from build123d import *

# Parameters (mm, degrees)
F1_R      = 46
F2_DEPTH  = 8
F3_R      = 39.8466862326
F4_DEPTH  = 6
F7_DEPTH  = 25
F9_ANGLE  = 120
F10_ANGLE = 120
F13_DEPTH = 8
F15_DEPTH = 8
F16_ANGLE = 120
F18_DEPTH = 6
F20_DEPTH = 6
F21_R     = 1
F22_R     = 2
F23_R     = 2


with BuildPart() as f2:
    # F1 (on offset) → F2 (new body)
    with BuildSketch(Plane.XY.offset(-3)):
        Circle(F1_R)
    extrude(amount=F2_DEPTH)


with BuildPart() as f4:
    # F3 (on Top) → F4 (new body)
    with BuildSketch(Plane.XY):
        Circle(F3_R)
    extrude(amount=F4_DEPTH)


with BuildPart() as f2_1:
    add(f2.part)

    # F5: cut F4
    add(f4.part, mode=Mode.SUBTRACT)


with BuildPart() as f7:
    # F6 (on Top) → F7 (new body)
    with BuildSketch(Plane.XY):
        Polygon((4.2, 46.7533776755), (-4.2, 46.7533776755), (-5, 38), (5, 38), align=None)
    extrude(amount=F7_DEPTH)


with BuildPart() as f9_1:
    # F9: copy of F7
    add(f7.part.rotate(Axis((0, 0, 3.5398988872), (0, 0, -1)), F9_ANGLE))


with BuildPart() as f10_1:
    # F10: copy of F9_1
    add(f9_1.part.rotate(Axis((0, 0, 3.5398988872), (0, 0, -1)), F10_ANGLE))


with BuildPart() as f2_2:
    add(f2_1.part)

    # F11: cut F10_1, F9_1, F7
    add(f10_1.part, mode=Mode.SUBTRACT)
    add(f9_1.part, mode=Mode.SUBTRACT)
    add(f7.part, mode=Mode.SUBTRACT)



with BuildPart() as f13:
    # F12 (on offset) → F13 (new body)
    with BuildSketch(Plane.XY.offset(-3)):
        Polygon((1.9, 49.994420498), (-1.9, 49.925893195), (-3, 36.9057094163), (3, 36.9057094163), align=None)
    extrude(amount=F13_DEPTH)


with BuildPart() as f15:
    # F14 (on offset) → F15 (new body)
    with BuildSketch(Plane.XY.offset(-3)):
        Polygon((42.1813093126, -26.4778193086), (44.179931283, -23.2300590724), (28.5657010972, -12.1127264574), (24.8182862997, -18.1085914373), align=None)
    extrude(amount=F15_DEPTH)


with BuildPart() as f16_1:
    # F16: copy of F15
    add(f15.part.rotate(Axis((0, 0, 3.5398988872), (0, 0, -1)), F16_ANGLE))


with BuildPart() as f18:
    # F17 (on Top) → F18 (new body)
    with BuildSketch(Plane.XY):
        Polygon((25.2, 21.096765488), (12.9, 34.6466732368), (-12.9, 34.6466732368), (-25.2, 21.096765488), (-24.2, 6.7315296738), (-30.2, 5.9), (-30.2, -2.6), (-25.2, -4.6), (-21, -5.2), (-21, 3.5), (-3.3, -0.8), (3.3, -0.8), (21, 3.5), (21, -5.2), (25.2, -4.6), (30.2, -2.5974751513), (30.2, 5.9025248487), (24.2, 6.7315296738), align=None)
    extrude(amount=F18_DEPTH)


with BuildPart() as f2_3:
    add(f2_2.part)

    add(f13.part)  # F20 merges F13

    add(f15.part)  # F20 merges F15

    add(f16_1.part)  # F20 merges F16_1

    add(f18.part)  # F20 merges F18
    # F19 (on Top) → F20 (join)
    with BuildSketch(Plane.XY):
        Polygon((3.1, -11), (0, -7.4), (-3.1, -11), (-15.2, -11), (-20.6, -8), (-24.6, -7.5), (-26.5, -9.7), (-21.4, -17.7), (-17, -18), (-15, -18.5), (-11, -21.7), (-14, -29.7), (-9.8, -33.1), (-8, -31.2), (-6.6, -34.4), (-1.4, -35.8), (-0.5, -21), (-3.8, -22.2), (0, -14), (3.8, -22.2), (0.5, -21), (1.4, -35.8), (6.6, -34.4), (8, -31.2), (9.8, -33.1), (14, -29.7), (11, -21.7), (15, -18.5), (17, -18), (21.4, -17.7), (26.5, -9.7), (24.6, -7.5), (20.6, -8), (15.2, -11), align=None)
    extrude(amount=F20_DEPTH)

    # F21
    f21_edges = [f2_3.edges().sort_by_distance(p)[0] for p in [
        (1.9, 49.99442, 1),
        (-1.9, 49.925893, 1),
        (3, 36.905709, 2.5),
        (-3, 36.905709, 2.5),
        (-28.091643, -12.438971, 2.5),
        (-44.021119, -23.291176, 1),
        (-42.207787, -26.645913, 1),
        (-24.772779, -18.68226, 2.5),
        (24.818286, -18.108591, 2.5),
        (28.565701, -12.112726, 2.5),
        (42.181309, -26.477819, 1),
        (44.179931, -23.230059, 1),
        (37.520202, -26.612675, 2.5),
        (41.807353, -19.18711, 2.5),
        (36.679976, -15.567202, 2.5),
        (31.82158, -23.98219, 2.5),
        (4.287152, 45.799785, 2.5),
        (-4.287152, 45.799785, 2.5),
        (-4.858396, 39.549392, 2.5),
        (4.858396, 39.549392, 2.5),
        (-41.807353, -19.18711, 2.5),
        (-37.520202, -26.612675, 2.5),
        (-36.679976, -15.567202, 2.5),
        (-31.82158, -23.98219, 2.5),
    ]]
    fillet(f21_edges, radius=F21_R)

    # F22
    f22_edges = [f2_3.edges().sort_by_distance(p)[0] for p in [
        (30.2, 5.902525, 3),
        (30.2, -2.597475, 3),
        (24.2, 6.73153, 3),
        (25.2, 21.096765, 3),
        (12.9, 34.646673, 3),
        (-12.9, 34.646673, 3),
        (-25.2, 21.096765, 3),
        (-24.2, 6.73153, 3),
        (-30.2, 5.9, 3),
        (-30.2, -2.6, 3),
        (-25.2, -4.6, 3),
        (-21, -5.2, 3),
        (-21, 3.5, 3),
        (-3.3, -0.8, 3),
        (3.3, -0.8, 3),
        (21, 3.5, 3),
        (21, -5.2, 3),
        (25.2, -4.6, 3),
    ]]
    fillet(f22_edges, radius=F22_R)

    # F23
    f23_edges = [f2_3.edges().sort_by_distance(p)[0] for p in [
        (26.5, -9.7, 3),
        (21.4, -17.7, 3),
        (17, -18, 3),
        (15, -18.5, 3),
        (11, -21.7, 3),
        (-11, -21.7, 3),
        (-15, -18.5, 3),
        (-17, -18, 3),
        (-21.4, -17.7, 3),
        (-26.5, -9.7, 3),
        (-24.6, -7.5, 3),
        (-20.6, -8, 3),
        (-15.2, -11, 3),
        (-3.1, -11, 3),
        (3.1, -11, 3),
        (15.2, -11, 3),
        (20.6, -8, 3),
        (24.6, -7.5, 3),
    ]]
    fillet(f23_edges, radius=F23_R)


with BuildPart() as f24_1:
    # F24: copy of F2
    add(f2_3.part)


solid = f2_3.part
Verification items for the finished model (mm, model axes). A direction names the side the tool comes from. Coordinates: 2 decimals unless noted, no trailing zeros. Order: outer loops, then holes, each group sorted by start corner. A loop starts at its lowest first (then second) coordinate and runs counter-clockwise, first axis right, second up.
Item 1: Access from +Z, -Z, +X, -X, +Y, -Y to the whole of each face (thin tool, end or side, straight path). Record for faces 1 (the face through (34, -19, 5)), 2 (the face through (0, 44, 5)), 3 (the face through (12.772, -26.425, 2.958)).
Filled in:
face 1: +Z, +X, -Y
face 2: +Z, +X, -X, +Y
face 3: +Z
Item 2: Section check B-B, the plane z = 3. Give the number of separate pieces and of enclosed holes in the cut face, then the cut area to 3 significant figures.
Filled in:
separate pieces: 8
enclosed holes: 0
area: 4,160 mm2
Item 3: Section check A-A, the plane y = 17. Enter the section's corners in (x, z).
Filled in:
outline: (-42.74, -3) - (42.74, -3) - (42.74, 5) - (36.04, 5) - (36.04, 0) - (24.91, 0) - (24.91, 6) - (-24.91, 6) - (-24.91, 0) - (-36.04, 0) - (-36.04, 5) - (-42.74, 5) - close
Item 4: Material ranges on L1, parallel to X at y = -29, z = 1.25; L2, parallel to Y at x = -9.5, z = 1.75; L3, parallel to Y at x = 11, z = 1.5, recorded low to high.
Filled in:
L1: x = -35.71 to -27.33, -13.74 to -0.99, 0.99 to 13.74, 27.33 to 35.71
L2: y = -45.01 to -38.7, -32.78 to -11, 0.71 to 34.65, 38.7 to 45.01
L3: y = -44.67 to -38.3, -32.13 to -11, 1.07 to 34.65, 38.3 to 44.67
Item 5: Section check C-C, the plane y = 42.5. Enter the section's corners in (x, z), then the cut area to 3 significant figures.
Filled in:
outline: (-17.6, -3) - (17.6, -3) - (17.6, 5) - (4.59, 5) - (4.59, 0) - (2.53, 0) - (2.53, 5) - (-2.53, 5) - (-2.53, 0) - (-4.59, 0) - (-4.59, 5) - (-17.6, 5) - close
area: 261 mm2
Item 6: Depth check by flat-ended pin: pin 1 (5 mm diameter, centred on x = -1, z = 2.5, fed in from +Y); pin 2 (1 mm diameter, centred on y = -3.5, z = 4, fed in from -X); pin 3 (1 mm diameter, centred on x = -14, z = 2.5, fed in from -Y); pin 4 (1.5 mm diameter, centred on y = 4.5, z = -2, fed in from +X). Enter the tip coordinate at first touch or a pass-through.
Filled in:
pin 1: stops at y = 49.98
pin 2: stops at x = -45.9
pin 3: stops at y = -43.97
pin 4: stops at x = 45.85
